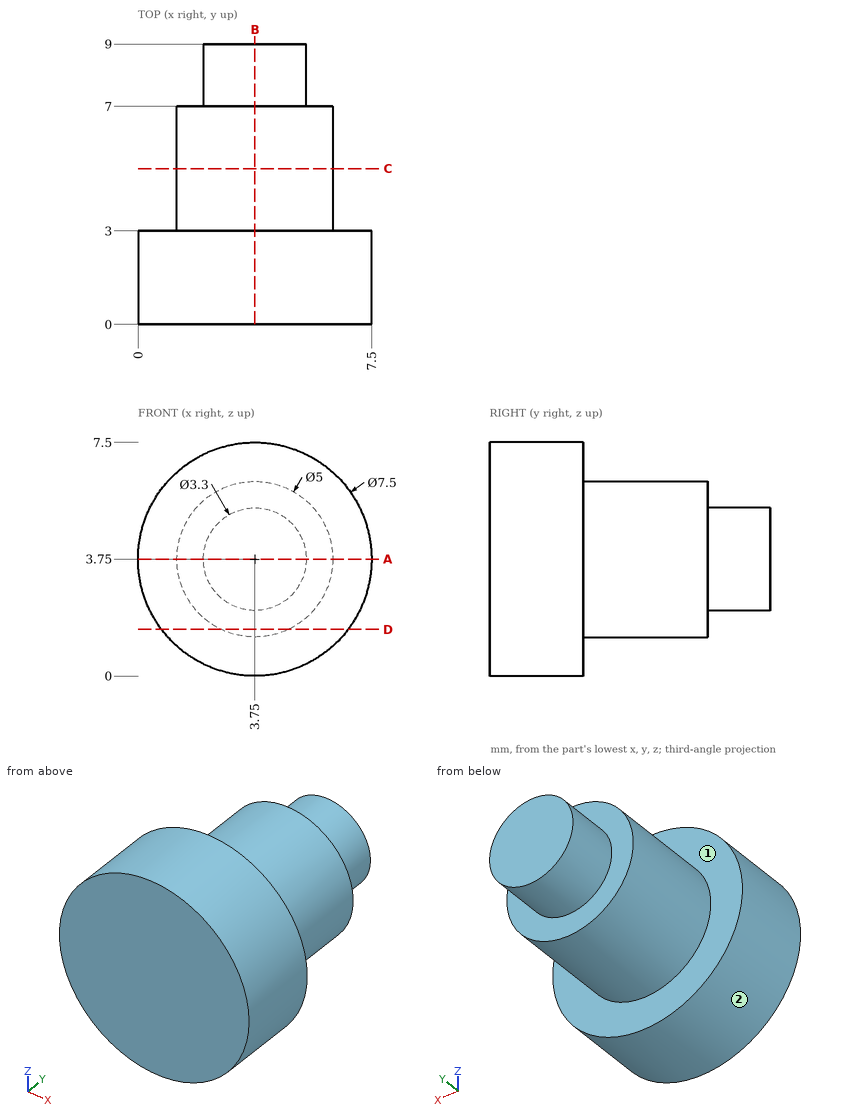
Verification items for this drawing (mm, ordinates from the low corner). A direction names the side the tool comes from. Coordinates: 2 decimals unless noted, no trailing zeros. Order: outer loops, then holes, each group sorted by start corner. A loop starts at its lowest first (then second) coordinate and runs counter-clockwise, first axis right, second up. Notation, with made-up numbers: (0.25, -15.5) - (37.25, -15.5) arc R18 cw to (37.25, 2.5) - close; hole circle Ø9 at (41.5, -13.75). An arc over 180 degrees is marked (long way). Use one line per item in the form item = value.
1. Section check B-B (x = 3.75). Record the boundary of the cut face in (y, z), then the cut area to 3 significant figures.
Here are the results:
outline = (0, 0) - (3, 0) - (3, 1.25) - (7, 1.25) - (7, 2.1) - (9, 2.1) - (9, 5.4) - (7, 5.4) - (7, 6.25) - (3, 6.25) - (3, 7.5) - (0, 7.5) - close
area = 49.1 mm²
2. Access from +Z, -Z, +X, -X, +Y, -Y to the whole of each face (thin tool, end or side, straight path). Record for the marked faces 1 and 2.
Here are the results:
face_1 = +Y
face_2 = +Y, -Y
3. Section check D-D (z = 1.5). Record the boundary of the cut face in (x, y).
Here are the results:
outline = (0.75, 0) - (6.75, 0) - (6.75, 3) - (4.84, 3) - (4.84, 7) - (2.66, 7) - (2.66, 3) - (0.75, 3) - close
4. Scan lines: line 1 (Y direction, x = 2, z = 4); line 2 (Y direction, x = 6, z = 5); line 3 (Z direction, x = 3, y = 1). Record each from-to range of solid material in increasing order.
Here are the results:
line_1 = 0 to 7
line_2 = 0 to 3
line_3 = 0.08 to 7.42
5. Section check C-C (y = 5). Record the boundary of the cut face in (x, z), then the cut area to 3 significant figures.
Here are the results:
outline = circle Ø5 at (3.75, 3.75)
area = 19.6 mm²
6. Section check A-A (z = 3.75). Record the boundary of the cut face in (x, y), then the cut area to 3 significant figures.
Here are the results:
outline = (0, 0) - (7.5, 0) - (7.5, 3) - (6.25, 3) - (6.25, 7) - (5.4, 7) - (5.4, 9) - (2.1, 9) - (2.1, 7) - (1.25, 7) - (1.25, 3) - (0, 3) - close
area = 49.1 mm²
